```python
from build123d import *

# Parameters (mm, degrees)
F0_R     = 60
F0_R_2   = 5
F1_DEPTH = 20


with BuildPart() as f1:
    # F0 (on Front) → F1 (new body)
    with BuildSketch(Plane.XZ):
        Circle(F0_R)
        with Locations((-35.355339, -35.355339)):
            Circle(F0_R_2, mode=Mode.SUBTRACT)
        with Locations((0, -50)):
            Circle(F0_R_2, mode=Mode.SUBTRACT)
        with Locations((35.355339, -35.355339)):
            Circle(F0_R_2, mode=Mode.SUBTRACT)
        with Locations((-50, 0)):
            Circle(F0_R_2, mode=Mode.SUBTRACT)
        with Locations((-35.355339, 35.355339)):
            Circle(F0_R_2, mode=Mode.SUBTRACT)
        with Locations((50, 0)):
            Circle(F0_R_2, mode=Mode.SUBTRACT)
        with Locations((0, 50)):
            Circle(F0_R_2, mode=Mode.SUBTRACT)
        with Locations((35.355339, 35.355339)):
            Circle(F0_R_2, mode=Mode.SUBTRACT)
    extrude(amount=F1_DEPTH)

    # F2 (on Top) → F3 (revolve)
    with BuildSketch(Plane.XY):
        with BuildLine():
            Line((-40, 0), (0, 0))
            Line((0, 0), (0, 40))
            ThreePointArc((0, 40), (-28.284271, 28.284271), (-40, 0))
        make_face()
    revolve(axis=Axis((0, 20, 0), (0, 1, 0)))


solid = f1.part
```
CAD build for the part. Positions are in the model's coordinates, mm. Round coordinates to 2 decimals unless told otherwise and drop trailing zeros. Write each loop counter-clockwise with the first axis right and the second up, starting at its lowest first coordinate (ties: lowest second). Pieces come first, ordered by that corner, then holes. Notation, with made-up numbers: (-39, 22.5) - (-23, 22.5) arc R24 cw to (-23, 47.5) - close; hole circle Ø4 at (10.25, 55.25). An arc over 180 degrees is marked (long way). Return JSON: item names as keys, results as strings. Group by question number.
Item 1: Probe probe 1 along X at (y, z) = (-6, 0.5); probe 2 along Z at (x, y) = (-32.5, -2); probe 3 along Y at (x, z) = (-41.5, 28). List the from-to ranges inside material, lowest first.
Item 2: Flat gauge pins, fed straight in: pin 1 Ø6 at (y, z) = (-14, 21) entering from +X; pin 2 Ø16 at (x, z) = (0, 50) entering from -Y; pin 3 Ø1 at (x, z) = (19, 8) entering from +Y; pin 4 Ø11.5 at (x, z) = (35.36, -35.36) entering from +Y. Where does each tip first touch, or does it go through?
Item 3: Band-saw the part on C-C on y = -8.5. State how many separate pieces and enclosed holes the cut face has, plus the area to 3 significant figures.
Item 4: Band-saw the part on A-A on z = 50. List the corners of the cut face in (x, y), plus the area to 3 significant figures.
Item 5: Band-saw the part on B-B on x = -50. List the corners of the cut face in (y, z).
Item 6: Mould opens along X. For faces 1 (the face through (-39.041, -9.86, -31.976)), 2 (the face through (-59.94, -9.86, 2.64)), 3 (the face through (-0.651, -9.86, 54.957)), 4 (the face through (12, 0, -39)) say: +X half, -X half, draft (parallel to the pull), parting line (faces both ways), or undercut.
Resolved:
{
 "1": {"probe 1": "x = -60 to -54.97, -45.03 to 45.03, 54.97 to 60", "probe 2": "z = -50.44 to -39.46, -31.25 to 31.25, 39.46 to 50.44", "probe 3": "y = -20 to 0"},
 "2": {"pin 1": "stops at x = 57.24", "pin 2": "stops at y = -20", "pin 3": "stops at y = 34.57", "pin 4": "stops at y = 0"},
 "3": {"separate pieces": "1", "enclosed holes": "8", "area": "10,700 mm²"},
 "4": {"outline": "(-33.17, -20) - (-5, -20) - (-5, 0) - (-33.17, 0) - close; (5, -20) - (33.17, -20) - (33.17, 0) - (5, 0) - close", "area": "1,130 mm²"},
 "5": {"outline": "(-20, -33.17) - (0, -33.17) - (0, -5) - (-20, -5) - close; (-20, 5) - (0, 5) - (0, 33.17) - (-20, 33.17) - close"},
 "6": {"face 1": "undercut", "face 2": "parting line", "face 3": "undercut", "face 4": "draft"}
}
